Check sheet for the modelled part. Datum: model origin and axes. Units: mm. Face numbers are marked on the shaded views. A direction names the side the tool comes from. Give positions to 0.01 mm unless a question says otherwise; leave off trailing zeros. Order: outer loops, then holes, each group sorted by start corner. A loop starts at its lowest first (then second) coordinate and runs counter-clockwise, first axis right, second up. Notation, with made-up numbers: (54, -23.75) -> (111, -23.75) arc R34 ccw to (111, 12.25) -> close; hole circle Ø7 at (52.5, 25). An arc over 180 degrees is marked (long way). Write each question's results on one line, items separated by ' | '.
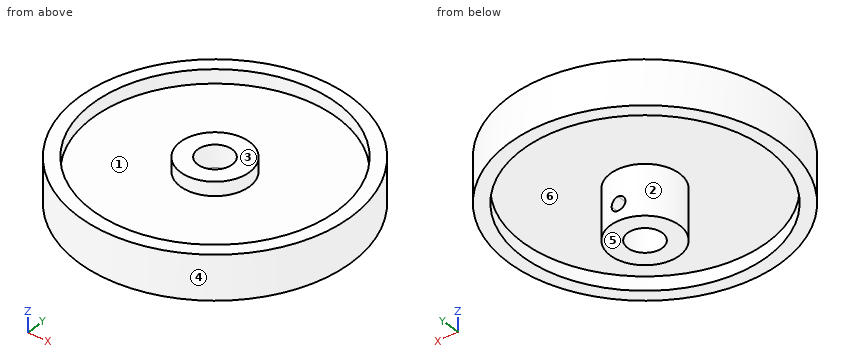
from build123d import *

# Parameters (mm, degrees)
F0_R          = 49.25
F0_R_2        = 44.25
F1_DEPTH      = 8
F0_R_3        = 12.5
F2_DEPTH      = 3
F0_R_4        = 6.25
F3_DEPTH      = 8
F3_DEPTH_BACK = 21
F5_DEPTH      = 25


with BuildPart() as f1:
    # F0 (on Top) → F1 (new body, symmetric)
    with BuildSketch(Plane.XY):
        Circle(F0_R)
        Circle(F0_R_2, mode=Mode.SUBTRACT)
    extrude(amount=F1_DEPTH, both=True)

    # F0 (on Top) → F2 (join, symmetric)
    with BuildSketch(Plane.XY):
        Circle(F0_R_2)
        Circle(F0_R_3, mode=Mode.SUBTRACT)
    extrude(amount=F2_DEPTH, both=True)

    # F0 (on Top) → F3 (join, two sides)
    with BuildSketch(Plane.XY) as f3_sk:
        Circle(F0_R_3)
        Circle(F0_R_4, mode=Mode.SUBTRACT)
    extrude(amount=F3_DEPTH)
    extrude(f3_sk.sketch, amount=-F3_DEPTH_BACK)

    # F4 (on Front) → F5 (cut)
    with BuildSketch(Plane.XZ):
        with BuildLine():
            ThreePointArc((0, -12.5), (-1.767767, -16.767767), (2.5, -15))
            ThreePointArc((2.5, -15), (1.767767, -13.232233), (0, -12.5))
        make_face()
    extrude(amount=-F5_DEPTH, mode=Mode.SUBTRACT)


solid = f1.part
1. Material ranges on probe 1 along Y at (x, z) = (0, 4.7); probe 2 along Y at (x, z) = (-5, 5.25); probe 3 along Z at (x, y) = (-26.5, -25), recorded low to high. Write a range as from..to.
Verdict:
probe 1: y = -49.25..-44.25, -12.5..-6.25, 6.25..12.5, 44.25..49.25 | probe 2: y = -49..-43.97, -11.46..-3.75, 3.75..11.46, 43.97..49 | probe 3: z = -3..3
2. Section check D-D on x = 31. Record the cut outline in (y, z), then the cut area to 3 significant figures.
Verdict:
outline: (-38.27, -8) -> (-31.58, -8) -> (-31.58, -3) -> (31.58, -3) -> (31.58, -8) -> (38.27, -8) -> (38.27, 8) -> (31.58, 8) -> (31.58, 3) -> (-31.58, 3) -> (-31.58, 8) -> (-38.27, 8) -> close | area: 593 mm^2
3. Section check C-C on z = 1.25. Record the cut outline in (x, y).
Verdict:
outline: circle Ø98.5 at (0, 0); hole circle Ø12.5 at (0, 0)
4. Access from +Z, -Z, +X, -X, +Y, -Y to the whole of each face (thin tool, end or side, straight path). Record for the marked faces 1, 2 and 3.
Verdict:
face 1: +Z | face 2: -Z | face 3: +Z, +X, -X, +Y, -Y
5. Section check A-A on y = 0. Record the cut outline in (x, z).
Verdict:
outline: (-49.25, -8) -> (-44.25, -8) -> (-44.25, -3) -> (-12.5, -3) -> (-12.5, -21) -> (-6.25, -21) -> (-6.25, 8) -> (-12.5, 8) -> (-12.5, 3) -> (-44.25, 3) -> (-44.25, 8) -> (-49.25, 8) -> close; (6.25, -21) -> (12.5, -21) -> (12.5, -3) -> (44.25, -3) -> (44.25, -8) -> (49.25, -8) -> (49.25, 8) -> (44.25, 8) -> (44.25, 3) -> (12.5, 3) -> (12.5, 8) -> (6.25, 8) -> close
6. Mould release check, pull along X, two halves, no side actions. Record for the marked faces 4, 5 and 6: +X half, -X half, draft (parallel to the pull), parting line (faces both ways), or undercut.
Verdict:
face 4: parting line | face 5: draft | face 6: undercut
7. Gauge pin test, flat ends, axial feed: pin 1 Ø10 at (y, z) = (-15, 0) entering from -X; pin 2 Ø2 at (x, y) = (36.5, 17) entering from +Z; pin 3 Ø4 at (x, y) = (9.5, 22.5) entering from -Z. Record the tip position at first contact, or that the pin passes through.
Verdict:
pin 1: stops at x = -48.22 | pin 2: stops at z = 3 | pin 3: stops at z = -3
8. Section check B-B on z = -5.75. Record the cut outline in (x, y).
Verdict:
outline: circle Ø98.5 at (0, 0); circle Ø25 at (0, 0); hole circle Ø88.5 at (0, 0); hole circle Ø12.5 at (0, 0)
